Source: CAD feature listing. Evaluate the final solid. Frame: model axes, mm. Give positions to 0.01 mm unless a question says otherwise; leave off trailing zeros. Order: outer loops, then holes, each group sorted by start corner. A loop starts at its lowest first (then second) coordinate and runs counter-clockwise, first axis right, second up.
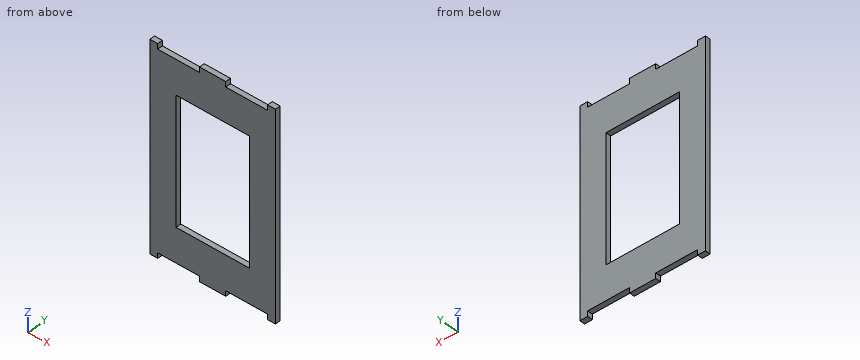
```python
from build123d import *

# Parameters (mm, degrees)
ESQUISSE1_W        = 140
ESQUISSE1_H        = 240
BOSS_EXTRU_1_DEPTH = 10


with BuildPart() as part:
    # Esquisse1 → Boss.-Extru.1 (new body)
    with BuildSketch(Plane(origin=(0, 0, 0), x_dir=(1, 0, 0), z_dir=(0, 1, 0))):
        Polygon((15, 10), (15, 0), (0, 0), (0, 10), (0, 380), (0, 390), (15, 390), (15, 380), (95, 380), (95, 390), (145, 390), (145, 380), (225, 380), (225, 390), (240, 390), (240, 380), (240, 10), (240, 0), (225, 0), (225, 10), (145, 10), (145, 0), (95, 0), (95, 10), align=None)
        with Locations((120, 195)):
            Rectangle(ESQUISSE1_W, ESQUISSE1_H, mode=Mode.SUBTRACT)
    extrude(amount=BOSS_EXTRU_1_DEPTH)


solid = part.part
```
1) Section query A-A, the plane x = 128. Return the cut outline in (y, z), and give its area (3 significant figures).
Report:
outline: (0, -390) - (10, -390) - (10, -315) - (0, -315) - close; (0, -75) - (10, -75) - (10, 0) - (0, 0) - close
area: 1,500 mm2
2) Section query B-B, the plane y = 2.75. Return the cut outline in (x, z).
Report:
outline: (0, -390) - (15, -390) - (15, -380) - (95, -380) - (95, -390) - (145, -390) - (145, -380) - (225, -380) - (225, -390) - (240, -390) - (240, 0) - (225, 0) - (225, -10) - (145, -10) - (145, 0) - (95, 0) - (95, -10) - (15, -10) - (15, 0) - (0, 0) - close; hole (50, -315) - (190, -315) - (190, -75) - (50, -75) - close
3) Section query C-C, the plane z = -237. Return the cut outline in (x, y).
Report:
outline: (0, 0) - (50, 0) - (50, 10) - (0, 10) - close; (190, 0) - (240, 0) - (240, 10) - (190, 10) - close
4) Pin query (flat end, axial travel): pin 1 (2 mm diameter, centred on x = 40.5, y = 1.5, fed in from +Z); pin 2 (5 mm diameter, centred on x = 188, y = 6.5, fed in from -Z). Return the tip coordinate at first contact, or that it passes through.
Report:
pin 1: stops at z = -10
pin 2: stops at z = -380
5) Section query D-D, the plane x = 217.5. Return the cut outline in (y, z).
Report:
outline: (0, -380) - (10, -380) - (10, -10) - (0, -10) - close
6) Material intervals for L1, parallel to Z at x = 182.5, y = 3; L2, parallel to X at y = 3, z = -92.5; L3, parallel to Z at x = 107.5, y = 2.75, sorted ascending.
Report:
L1: z = -380 to -315, -75 to -10
L2: x = 0 to 50, 190 to 240
L3: z = -390 to -315, -75 to 0
